from build123d import *

# Parameters (mm, degrees)
CYLINDER014005832_R     = 2.2
CYLINDER014005832_DEPTH = 200
CYLINDER014005833_R     = 2.2
CYLINDER014005833_DEPTH = 200
BOX138_W                = 9
BOX138_H                = 28
BOX138_DEPTH            = 20
BOX136_W                = 9
BOX136_H                = 28
BOX136_DEPTH            = 20
CYLINDER014005829_R     = 5.6
CYLINDER014005829_DEPTH = 4
CYLINDER014005827_R     = 2.7
CYLINDER014005827_DEPTH = 200
CYLINDER014005826_R     = 19
CYLINDER014005826_DEPTH = 20
CYLINDER014005828_R     = 3.2
CYLINDER014005828_DEPTH = 200
CYLINDER014005830_R     = 5.6
CYLINDER014005830_DEPTH = 4
BOX119_W                = 60
BOX119_H                = 52
BOX119_DEPTH            = 20
CHAMFER019_SIZE         = 10
BOX135_W                = 34
BOX135_H                = 14
BOX135_DEPTH            = 40
CHAMFER015_SIZE         = 7


with BuildPart() as obj1:
    # Cylinder014005832 → Cylinder014005832 (new body)
    with BuildSketch(Plane(origin=(-26, -22, -140), x_dir=(1, 0, 0), z_dir=(0, 0, 1))):
        Circle(CYLINDER014005832_R)
    extrude(amount=CYLINDER014005832_DEPTH)


with BuildPart() as fusion435:
    # Cylinder014005833 → Cylinder014005833 (new body)
    with BuildSketch(Plane(origin=(26, -22, -140), x_dir=(1, 0, 0), z_dir=(0, 0, 1))):
        Circle(CYLINDER014005833_R)
    extrude(amount=CYLINDER014005833_DEPTH)

    # Fusion435: union obj1
    add(obj1.part)


with BuildPart() as krychle125:
    # Box138 → Box138 (new body)
    with BuildSketch(Plane(origin=(21, -35, -81), x_dir=(1, 0, 0), z_dir=(0, 0, 1))):
        with Locations((4.5, 14)):
            Rectangle(BOX138_W, BOX138_H)
    extrude(amount=BOX138_DEPTH)


with BuildPart() as krychle123:
    # Box136 → Box136 (new body)
    with BuildSketch(Plane(origin=(-30, -35, -81), x_dir=(1, 0, 0), z_dir=(0, 0, 1))):
        with Locations((4.5, 14)):
            Rectangle(BOX136_W, BOX136_H)
    extrude(amount=BOX136_DEPTH)


with BuildPart() as obj2:
    # Cylinder014005829 → Cylinder014005829 (new body)
    with BuildSketch(Plane(origin=(0, -29, -97), x_dir=(1, 0, 0), z_dir=(0, 0, 1))):
        Circle(CYLINDER014005829_R)
    extrude(amount=CYLINDER014005829_DEPTH)


with BuildPart() as obj3:
    # Cylinder014005827 → Cylinder014005827 (new body)
    with BuildSketch(Plane(origin=(0, -29, -200), x_dir=(1, 0, 0), z_dir=(0, 0, 1))):
        Circle(CYLINDER014005827_R)
    extrude(amount=CYLINDER014005827_DEPTH)


with BuildPart() as obj4:
    # Cylinder014005826 → Cylinder014005826 (new body)
    with BuildSketch(Plane.XY.offset(-113)):
        Circle(CYLINDER014005826_R)
    extrude(amount=CYLINDER014005826_DEPTH)


with BuildPart() as obj5:
    # Cylinder014005828 → Cylinder014005828 (new body)
    with BuildSketch(Plane(origin=(0, -56, -200), x_dir=(1, 0, 0), z_dir=(0, 0, 1))):
        Circle(CYLINDER014005828_R)
    extrude(amount=CYLINDER014005828_DEPTH)


with BuildPart() as fusion442:
    # Cylinder014005830 → Cylinder014005830 (new body)
    with BuildSketch(Plane(origin=(0, -29, -113), x_dir=(1, 0, 0), z_dir=(0, 0, 1))):
        Circle(CYLINDER014005830_R)
    extrude(amount=CYLINDER014005830_DEPTH)

    # Fusion442: union obj2, obj3, obj4, obj5
    add(obj2.part)
    add(obj3.part)
    add(obj4.part)
    add(obj5.part)


with BuildPart() as chamfer019:
    # Box119 → Box119 (new body)
    with BuildSketch(Plane(origin=(-30, -49, -59), x_dir=(1, 0, 0), z_dir=(0, 0, 1))):
        with Locations((30, 26)):
            Rectangle(BOX119_W, BOX119_H)
    extrude(amount=BOX119_DEPTH)

    # Chamfer019
    chamfer019_edges = [chamfer019.edges().sort_by_distance(p)[0] for p in [
        (-30, -49, -49),
        (-30, 3, -49),
        (30, -49, -49),
        (30, 3, -49),
    ]]
    chamfer(chamfer019_edges, length=CHAMFER019_SIZE)


with BuildPart() as obj6:
    # Box135 → Box135 (new body)
    with BuildSketch(Plane(origin=(-17, -63, -59), x_dir=(1, 0, 0), z_dir=(0, 0, 1))):
        with Locations((17, 7)):
            Rectangle(BOX135_W, BOX135_H)
    extrude(amount=BOX135_DEPTH)

    # Chamfer015
    chamfer015_edges = [obj6.edges().sort_by_distance(p)[0] for p in [
        (-17, -63, -39),
        (17, -63, -39),
    ]]
    chamfer(chamfer015_edges, length=CHAMFER015_SIZE)

    # Fusion438: union Chamfer019
    add(chamfer019.part)


with BuildPart() as obj6_1:
    # Fusion438 placement: moved
    add(obj6.part.moved(Location((0, 0, -54))))

    # Cut061241: cut Fusion442
    add(fusion442.part, mode=Mode.SUBTRACT)


with BuildPart() as obj6_2:
    # Cut061241 placement: moved
    add(obj6_1.part.moved(Location((0, 0, 12))))

    # Fusion434: union Krychle125, Krychle123
    add(krychle125.part)
    add(krychle123.part)

    # Cut061305: cut Fusion435
    add(fusion435.part, mode=Mode.SUBTRACT)


with BuildPart() as obj6_3:
    # Cut061305 placement: moved
    add(obj6_2.part.moved(Location((0, 0, 2))))


solid = obj6_3.part
Input: part model. Units: mm. Frame: model coordinates. A direction names the side the tool comes from. Coordinates: 2 decimals unless noted, no trailing zeros. Write each loop counter-clockwise with the first axis right and the second up, starting at its lowest first coordinate (ties: lowest second). Pieces come first, ordered by that corner, then holes. Notation, with made-up numbers: M 38,70.5 L 65,70.5 A32 ccw 65,99.5 Z; hole C -33.75,59.25 d6. An arc over 180 degrees is marked long. Answer as a JSON object with one key per item and string values. Group by question number.
(1) Set-up query: faces 4 (the face through (25, -7, -69)), 5 (the face through (25, -35, -69)), 6 (the face through (-19, -49, -89)), 7 (the face through (18, -49, -89)). Return all of +Z, -Z, +X, -X, +Y, -Y with unobstructed straight access to the full face (end or side cutting, diameter ignored); none if empty.
(2) Section B-B on y = -22. Output: boundary loops of the cut face in (x, z), plus the area to 3 significant figures.
(3) Ray query, line 1 along X through (y, z) = (-22, -73); line 2 along X through (y, z) = (-34.5, -76.5); line 3 along X through (y, z) = (-2, -91). Return the intervals inside material, ascending. Write a range as [from, to].
(4) Contact query for flat-ended pins moving along their axis: P1, Ø7.5, axis at y = -52.5, z = -84.5, coming from the -X side; P2, Ø3.5, axis at x = 19, z = -85, coming from the -Y side; P3, Ø3, axis at y = -49, z = -65.5, coming from the -X side. Output: stop coordinate, or through.
(5) Mould query, pull axis X, two halves, no side actions, for faces 1 (the face through (23, -21, -59)), 2 (the face through (-30, -23, -79)), 3 (the face through (-1.214, -34.467, -81.028)). Classes: pulls with the +X half, pulls with the -X half, needs draft (parallel to the pull), parting line crosses it, or undercut.
(6) Section C-C on x = 26. Output: boundary loops of the cut face in (y, z).
(7) Section A-A on z = -63.5. Output: boundary loops of the cut face in (x, y).
(8) Section D-D on y = 0. Output: boundary loops of the cut face in (x, z).
Result set:
{
 "1": {"face 4": "+Z, +X, -X, +Y", "face 5": "+Z, +X, -X, -Y", "face 6": "+Z, -Z, -X, -Y", "face 7": "+Z, -Z, +X, -Y"},
 "2": {"outline": "M -30,-99 L -28.2,-99 L -28.2,-59 L -30,-59 Z; M -23.8,-99 L 23.8,-99 L 23.8,-59 L 21,-59 L 21,-79 L -21,-79 L -21,-59 L -23.8,-59 Z; M 28.2,-99 L 30,-99 L 30,-59 L 28.2,-59 Z", "area": "1,210 mm2"},
 "3": {"line 1": "x = [-30, -28.2], [-23.8, -21], [21, 23.8], [28.2, 30]", "line 2": "x = [-30, -21], [21, 30]", "line 3": "x = [-25, -18.89], [18.89, 25]"},
 "4": {"P1": "stops at x = -20.25", "P2": "stops at y = -49", "P3": "stops at x = -17"},
 "5": {"face 1": "needs draft", "face 2": "pulls with the -X half", "face 3": "undercut"},
 "6": {"outline": "M -43,-99 L -24.2,-99 L -24.2,-59 L -35,-59 L -35,-79 L -43,-79 Z; M -19.8,-99 L -3,-99 L -3,-79 L -7,-79 L -7,-59 L -19.8,-59 Z"},
 "7": {"outline": "M -30,-35 L -21,-35 L -21,-7 L -30,-7 Z; M -17,-56 L -10,-63 L 10,-63 L 17,-56 L 17,-49 L -17,-49 Z; M 21,-35 L 30,-35 L 30,-7 L 21,-7 Z; hole C -26,-22 d4.4; hole C 0,-56 d6.4; hole C 26,-22 d4.4"},
 "8": {"outline": "M -23,-99 L -19,-99 L -19,-79 L -23,-79 Z; M 19,-99 L 23,-99 L 23,-79 L 19,-79 Z"}
}
